Part model, mm, in its own coordinate system. A direction names the side the tool comes from. Coordinates: 2 decimals unless noted, no trailing zeros. Loops run counter-clockwise (first coordinate to the right, second up) from the corner with the lowest first, then second, coordinate; pieces in that order, holes last. Notation, with made-up numbers: M 56,63 L 107,63 A19 ccw 107,96 Z; hole C 58,50.5 d5. An arc over 180 degrees is marked long. Answer as a JSON object with one key per item and string values. Group by question number.
1. Saw through at C-C on z = -21577. Write the cut outline in (x, y), then the cut area to 3 significant figures.
2. Saw through at A-A on y = 40754.5. Count the separate pieces of the cut face and the enclosed holes in it, then the cut area to 3 significant figures.
3. Drill centre lines: L1, parallel to X at y = 40653, z = -21672.5; L2, parallel to Z at x = -11417, y = 40748; L3, parallel to Z at x = -11296, y = 40755. Where is each one in solid material? Low to high.
4. Drop flat-ended pins along their axis: pin 1 Ø3 at (x, y) = (-11272, 40756) entering from +Z; pin 2 Ø2.5 at (y, z) = (40753, -21693) entering from +X; pin 3 Ø2.5 at (x, y) = (-11252.5, 40751) entering from -Z. Give the stop position or say it passes through.
5. 3-axis set-ups, long thin cutter, end or side, ignore diameter. For faces 4 (the face through (-11340, 40808.218, -21603)), 5 (the face through (-11380.35, 40670.4, -21648.27)), 6 (the face through (-11327.54, 40686.12, -21589.43)): which of +Z, -Z, +X, -X, +Y, -Y reach the whole face in a straight line?
6. Mould opens along Y. For faces 1 (the face through (-11340, 40558.218, -21603)), 2 (the face through (-11343.109, 40684.968, -21599.265)), 3 (the face through (-11327.477, 40790.317, -21589.369)) say: released by +Y, released by -Y, zero draft, split by the parting line, or undercut.
7. Saw through at B-B on y = 40603. Write the cut outline in (x, z), then the cut area to 3 significant figures.
from build123d import *

# Parameters (mm, degrees)
SKETCH1_W               = 285
SKETCH1_H               = 250
BOSS_EXTRUDE1_DEPTH     = 10
CUT_EXTRUDE1_DEPTH      = 143.5
CUT_EXTRUDE1_DEPTH_BACK = 153.5
CHAMFER1_SIZE           = 2
SKETCH6_R               = 3.35
CUT_EXTRUDE4_DEPTH      = 153.5


with BuildPart() as part:
    # Sketch1 → Boss-Extrude1 (new body)
    with BuildSketch(Plane(origin=(5128.077990588, 0, -5128.077990588), x_dir=(-0.707106781, 0, -0.707106781), z_dir=(0.707106781, 0, -0.707106781))):
        with Locations((23295.770603259, 40683.217604407)):
            Rectangle(SKETCH1_W, SKETCH1_H)
    extrude(amount=BOSS_EXTRUDE1_DEPTH)

    # Sketch2 → Cut-Extrude1 (cut, two sides)
    with BuildSketch(Plane(origin=(5135.1490584, 0, -5135.1490584), x_dir=(-0.707106781, 0, -0.707106781), z_dir=(0.707106781, 0, -0.707106781))) as cut_extrude1_sk:
        with BuildLine():
            Line((23183.870603259, 40788.217604407), (23183.870603259, 40674.717604407))
            ThreePointArc((23183.870603259, 40674.717604407), (23179.870603259, 40670.717604407), (23175.870603259, 40674.717604407))
            Line((23175.870603259, 40674.717604407), (23175.870603259, 40788.217604407))
            ThreePointArc((23175.870603259, 40788.217604407), (23179.870603259, 40792.217604407), (23183.870603259, 40788.217604407))
        make_face()
        with BuildLine():
            Line((23358.670603259, 40788.217604407), (23358.670603259, 40674.717604407))
            ThreePointArc((23358.670603259, 40674.717604407), (23354.670603259, 40670.717604407), (23350.670603259, 40674.717604407))
            Line((23350.670603259, 40674.717604407), (23350.670603259, 40788.217604407))
            ThreePointArc((23350.670603259, 40788.217604407), (23354.670603259, 40792.217604407), (23358.670603259, 40788.217604407))
        make_face()
        with BuildLine():
            Line((23240.870603259, 40788.217604407), (23240.870603259, 40674.717604407))
            ThreePointArc((23240.870603259, 40674.717604407), (23236.870603259, 40670.717604407), (23232.870603259, 40674.717604407))
            Line((23232.870603259, 40674.717604407), (23232.870603259, 40788.217604407))
            ThreePointArc((23232.870603259, 40788.217604407), (23236.870603259, 40792.217604407), (23240.870603259, 40788.217604407))
        make_face()
        with BuildLine():
            Line((23415.670603259, 40788.217604407), (23415.670603259, 40674.717604407))
            ThreePointArc((23415.670603259, 40674.717604407), (23411.670603259, 40670.717604407), (23407.670603259, 40674.717604407))
            Line((23407.670603259, 40674.717604407), (23407.670603259, 40788.217604407))
            ThreePointArc((23407.670603259, 40788.217604407), (23411.670603259, 40792.217604407), (23415.670603259, 40788.217604407))
        make_face()
        with BuildLine():
            Line((23277.870603259, 40788.217604407), (23277.870603259, 40688.217604407))
            ThreePointArc((23277.870603259, 40688.217604407), (23275.770603259, 40686.117604407), (23273.670603259, 40688.217604407))
            Line((23273.670603259, 40688.217604407), (23273.670603259, 40788.217604407))
            ThreePointArc((23273.670603259, 40788.217604407), (23275.770603259, 40790.317604407), (23277.870603259, 40788.217604407))
        make_face()
        with BuildLine():
            Line((23313.670603259, 40788.217604407), (23313.670603259, 40688.217604407))
            ThreePointArc((23313.670603259, 40688.217604407), (23315.770603259, 40686.117604407), (23317.870603259, 40688.217604407))
            Line((23317.870603259, 40688.217604407), (23317.870603259, 40788.217604407))
            ThreePointArc((23317.870603259, 40788.217604407), (23315.770603259, 40790.317604407), (23313.670603259, 40788.217604407))
        make_face()
    extrude(amount=CUT_EXTRUDE1_DEPTH, mode=Mode.SUBTRACT)
    extrude(cut_extrude1_sk.sketch, amount=-CUT_EXTRUDE1_DEPTH_BACK, mode=Mode.SUBTRACT)

    # Chamfer1
    chamfer1_edges = [part.edges().sort_by_distance(p)[0] for p in [
        (-11323.306172507, 40790.317604407, -21593.604289307),
        (-11324.791096747, 40738.217604407, -21595.089213547),
        (-11323.306172507, 40686.117604407, -21593.604289307),
        (-11321.821248266, 40738.217604407, -21592.119365066),
        (-11419.40198407, 40792.217604407, -21689.70010087),
        (-11422.230411195, 40731.467604407, -21692.528527995),
        (-11419.40198407, 40670.717604407, -21689.70010087),
        (-11416.573556945, 40731.467604407, -21686.871673745),
        (-11379.096897542, 40792.217604407, -21649.395014342),
        (-11381.925324667, 40731.467604407, -21652.223441467),
        (-11379.096897542, 40670.717604407, -21649.395014342),
        (-11376.268470418, 40731.467604407, -21646.566587218),
        (-11295.799718719, 40792.217604407, -21566.097835519),
        (-11298.628145844, 40731.467604407, -21568.926262643),
        (-11295.799718719, 40670.717604407, -21566.097835519),
        (-11292.971291594, 40731.467604407, -21563.269408394),
        (-11351.590443754, 40790.317604407, -21621.888560554),
        (-11353.075367995, 40738.217604407, -21623.373484795),
        (-11351.590443754, 40686.117604407, -21621.888560554),
        (-11350.105519514, 40738.217604407, -21620.403636314),
        (-11255.494632191, 40792.217604407, -21525.792748991),
        (-11258.323059316, 40731.467604407, -21528.621176116),
        (-11255.494632191, 40670.717604407, -21525.792748991),
        (-11252.666205067, 40731.467604407, -21522.964321866),
    ]]
    chamfer(chamfer1_edges, length=CHAMFER1_SIZE)

    # Sketch6 → Cut-Extrude4 (cut, through all)
    with BuildSketch(Plane(origin=(5135.1490584, 0, -5135.1490584), x_dir=(-0.707106781, 0, -0.707106781), z_dir=(0.707106781, 0, -0.707106781))):
        with Locations((23320.047276205, 40623.466763723)):
            Circle(SKETCH6_R)
        with Locations((23280.047276205, 40623.466763723)):
            Circle(SKETCH6_R)
    extrude(amount=-CUT_EXTRUDE4_DEPTH, mode=Mode.SUBTRACT)


solid = part.part
Outcome:
{
 "1": {"outline": "M -11320.84,40558.22 L -11306.7,40558.22 L -11306.7,40808.22 L -11320.84,40808.22 Z", "area": "3,540 mm²"},
 "2": {"separate pieces": "7", "enclosed holes": "0", "area": "2,420 mm²"},
 "3": {"L1": "x = -11416.34 to -11402.2", "L2": "z = -21685.46 to -21673.16", "L3": "z = -21560.24 to -21552.16"},
 "4": {"pin 1": "stops at z = -21526.66", "pin 2": "stops at x = -11423.64", "pin 3": "stops at z = -21521.55"},
 "5": {"face 4": "+Z, -Z, +X, -X, +Y", "face 5": "-Z, +X", "face 6": "none"},
 "6": {"face 1": "released by -Y", "face 2": "zero draft", "face 3": "undercut"},
 "7": {"outline": "M -11445.28,-21701.44 L -11438.21,-21708.51 L -11236.69,-21506.98 L -11243.76,-21499.91 Z", "area": "2,850 mm²"}
}
